from build123d import *

# Parameters (mm, degrees)
CYLINDER001_R     = 15
CYLINDER001_DEPTH = 82
CYLINDER002_R     = 15
CYLINDER002_DEPTH = 82
CYLINDER003_R     = 15
CYLINDER003_DEPTH = 82
CYLINDER004_R     = 15
CYLINDER004_DEPTH = 82
CYLINDER005_R     = 15
CYLINDER005_DEPTH = 82
CYLINDER_R        = 15
CYLINDER_DEPTH    = 82
BOX_W             = 230
BOX_H             = 110
BOX_DEPTH         = 76


with BuildPart() as cilindre001:
    # Cylinder001 → Cylinder001 (new body)
    with BuildSketch(Plane(origin=(176, 76, -4), x_dir=(1, 0, 0), z_dir=(0, 0, 1))):
        Circle(CYLINDER001_R)
    extrude(amount=CYLINDER001_DEPTH)


with BuildPart() as cilindre002:
    # Cylinder002 → Cylinder002 (new body)
    with BuildSketch(Plane(origin=(176, 35, -4), x_dir=(1, 0, 0), z_dir=(0, 0, 1))):
        Circle(CYLINDER002_R)
    extrude(amount=CYLINDER002_DEPTH)


with BuildPart() as cilindre003:
    # Cylinder003 → Cylinder003 (new body)
    with BuildSketch(Plane(origin=(113, 76, -4), x_dir=(1, 0, 0), z_dir=(0, 0, 1))):
        Circle(CYLINDER003_R)
    extrude(amount=CYLINDER003_DEPTH)


with BuildPart() as cilindre004:
    # Cylinder004 → Cylinder004 (new body)
    with BuildSketch(Plane(origin=(52, 35, -4), x_dir=(1, 0, 0), z_dir=(0, 0, 1))):
        Circle(CYLINDER004_R)
    extrude(amount=CYLINDER004_DEPTH)


with BuildPart() as cilindre005:
    # Cylinder005 → Cylinder005 (new body)
    with BuildSketch(Plane(origin=(52, 76, -4), x_dir=(1, 0, 0), z_dir=(0, 0, 1))):
        Circle(CYLINDER005_R)
    extrude(amount=CYLINDER005_DEPTH)


with BuildPart() as cilindre:
    # Cylinder → Cylinder (new body)
    with BuildSketch(Plane(origin=(113, 35, -4), x_dir=(1, 0, 0), z_dir=(0, 0, 1))):
        Circle(CYLINDER_R)
    extrude(amount=CYLINDER_DEPTH)


with BuildPart() as cut005:
    # Box → Box (new body)
    with BuildSketch(Plane.XY):
        with Locations((115, 55)):
            Rectangle(BOX_W, BOX_H)
    extrude(amount=BOX_DEPTH)

    # Cut: cut Cilindre
    add(cilindre.part, mode=Mode.SUBTRACT)

    # Cut001: cut Cilindre005
    add(cilindre005.part, mode=Mode.SUBTRACT)

    # Cut002: cut Cilindre004
    add(cilindre004.part, mode=Mode.SUBTRACT)

    # Cut003: cut Cilindre003
    add(cilindre003.part, mode=Mode.SUBTRACT)

    # Cut004: cut Cilindre002
    add(cilindre002.part, mode=Mode.SUBTRACT)

    # Cut005: cut Cilindre001
    add(cilindre001.part, mode=Mode.SUBTRACT)


solid = cut005.part
Source: CAD feature listing. Evaluate the final solid. Frame: model axes, mm. Give positions to 0.01 mm unless a question says otherwise; leave off trailing zeros. Order: outer loops, then holes, each group sorted by start corner. A loop starts at its lowest first (then second) coordinate and runs counter-clockwise, first axis right, second up. Notation, with made-up numbers: (71.5, 56.25) -> (113.5, 56.25) arc R33 ccw to (113.5, 94.25) -> close; hole circle Ø11 at (56, -7.75). An arc over 180 degrees is marked (long way). Write item = value, one per line.
Item 1: Section query C-C (y = 76). Output: boundary loops of the cut face in (x, z), then the cut area to 3 significant figures.
Check result:
outline = (0, 0) -> (37, 0) -> (37, 76) -> (0, 76) -> close; (67, 0) -> (98, 0) -> (98, 76) -> (67, 76) -> close; (128, 0) -> (161, 0) -> (161, 76) -> (128, 76) -> close; (191, 0) -> (230, 0) -> (230, 76) -> (191, 76) -> close
area = 10,600 mm²
Item 2: Ray query, probe 1 along X at (y, z) = (76, 42); probe 2 along Y at (x, z) = (52, 21.5); probe 3 along X at (y, z) = (65, 4.5). Return the intervals inside material, ascending.
Check result:
probe_1 = 0 to 37, 67 to 98, 128 to 161, 191 to 230
probe_2 = 0 to 20, 50 to 61, 91 to 110
probe_3 = 0 to 41.8, 62.2 to 102.8, 123.2 to 165.8, 186.2 to 230
Item 3: Section query B-B (z = 21.5). Output: boundary loops of the cut face in (x, y), then the cut area to 3 significant figures.
Check result:
outline = (0, 0) -> (230, 0) -> (230, 110) -> (0, 110) -> close; hole circle Ø30 at (52, 35); hole circle Ø30 at (52, 76); hole circle Ø30 at (113, 35); hole circle Ø30 at (113, 76); hole circle Ø30 at (176, 35); hole circle Ø30 at (176, 76)
area = 21,100 mm²
Item 4: Mould query, pull axis X, two halves, no side actions, for faces 1 (the face through (48.748, 61.357, 37.468)), 2 (the face through (0, 54, 37)), 3 (the face through (113, 56, 76)). Classes: +X half, -X half, draft (parallel to the pull), parting line (faces both ways), or undercut.
Check result:
face_1 = undercut
face_2 = -X half
face_3 = draft
Item 5: Section query D-D (x = 125.5). Output: boundary loops of the cut face in (y, z), then the cut area to 3 significant figures.
Check result:
outline = (0, 0) -> (26.71, 0) -> (26.71, 76) -> (0, 76) -> close; (43.29, 0) -> (67.71, 0) -> (67.71, 76) -> (43.29, 76) -> close; (84.29, 0) -> (110, 0) -> (110, 76) -> (84.29, 76) -> close
area = 5,840 mm²
Item 6: Section query A-A (x = 52). Output: boundary loops of the cut face in (y, z).
Check result:
outline = (0, 0) -> (20, 0) -> (20, 76) -> (0, 76) -> close; (50, 0) -> (61, 0) -> (61, 76) -> (50, 76) -> close; (91, 0) -> (110, 0) -> (110, 76) -> (91, 76) -> close
Item 7: Contact query for flat-ended pins moving along their axis: pin 1 (10 mm diameter, centred on x = 33.5, z = 10.5, fed in from -Y); pin 2 (18 mm diameter, centred on x = 113, y = 35, fed in from -Z). Output: stop coordinate, or through.
Check result:
pin_1 = 0
pin_2 = through
